```python
from build123d import *

# Parameters (mm, degrees)
F0_W     = 139.7
F0_H     = 914.4
F1_DEPTH = 19.05
F2_W     = 139.7
F2_H     = 19.05
F3_DEPTH = 9.525


# Not quite as in the source:
# - a length typed as a fraction of an inch, garbled in the dataset ("3 / 203.2 mm" for 3/8 in), is restored


with BuildPart() as f1:
    # F0 (on Front) → F1 (new body)
    with BuildSketch(Plane.XZ):
        Rectangle(F0_W, F0_H)
    extrude(amount=F1_DEPTH)

    # F2 (on face) → F3 (cut)
    with BuildSketch(Plane(origin=(0, 0, 0), x_dir=(-1, 0, 0), z_dir=(0, 1, 0))):
        with Locations((0, 371.475)):
            Rectangle(F2_W, F2_H)
        with Locations((0, -3.175)):
            Rectangle(F2_W, F2_H)
        with Locations((0, -377.825)):
            Rectangle(F2_W, F2_H)
    extrude(amount=-F3_DEPTH, mode=Mode.SUBTRACT)


solid = f1.part
```
Build history of the part. All positions in model axes, mm. A direction names the side the tool comes from. Coordinates: 2 decimals unless noted, no trailing zeros. Order: outer loops, then holes, each group sorted by start corner. A loop starts at its lowest first (then second) coordinate and runs counter-clockwise, first axis right, second up.
Item 1: Drill centre lines: L1, parallel to Z at x = -12, y = -5; L2, parallel to Y at x = 8.5, z = -4.5 (3 decimals). Where is each one in solid material? Low to high.
Filled in:
L1: z = -457.2 to -387.35, -368.3 to -12.7, 6.35 to 361.95, 381 to 457.2
L2: y = -19.05 to -9.525
Item 2: Mould opens along Z. For faces 1 (the flat face through (-1, 0, 420)), 2 (the flat face through (1, -9.525, -378)), 3 (the flat face through (-1, -9, 457.2)), 4 (the flat face through (1, -9.525, 372)) say: released by +Z, released by -Z, zero draft, split by the parting line, or undercut.
Filled in:
face 1: zero draft
face 2: undercut
face 3: released by +Z
face 4: undercut
Item 3: Tool access for faces 5 (the flat face through (-1, 0, -188)), 6 (the flat face through (1, -9.525, -3)): list every direction of +Z, -Z, +X, -X, +Y, -Y with a clear straight run to the whole face (end or side of a thin tool).
Filled in:
face 5: +Z, -Z, +X, -X, +Y
face 6: +X, -X, +Y
Item 4: Saw through at A-A on x = -57. List the corners of the cut face in (y, z) (3 decimals).
Filled in:
outline: (-19.05, -457.2) - (0, -457.2) - (0, -387.35) - (-9.525, -387.35) - (-9.525, -368.3) - (0, -368.3) - (0, -12.7) - (-9.525, -12.7) - (-9.525, 6.35) - (0, 6.35) - (0, 361.95) - (-9.525, 361.95) - (-9.525, 381) - (0, 381) - (0, 457.2) - (-19.05, 457.2) - close
